```python
from build123d import *

# Parameters (mm, degrees)
SKETCH1_W           = 120
SKETCH1_H           = 200
BOSS_EXTRUDE1_DEPTH = 20
SKETCH2_W           = 120
SKETCH2_H           = 70
BOSS_EXTRUDE2_DEPTH = 15
SKETCH3_R           = 15
CUT_EXTRUDE1_DEPTH  = 119.321595662
FILLET1_R           = 40
CHAMFER1_SIZE       = 7
SHELL2_T            = -5


with BuildPart() as part:
    # Sketch1 → Boss-Extrude1 (new body)
    with BuildSketch(Plane.XY):
        Rectangle(SKETCH1_W, SKETCH1_H)
    extrude(amount=BOSS_EXTRUDE1_DEPTH)

    # Sketch2 → Boss-Extrude2 (add)
    with BuildSketch(Plane.XY.offset(20)):
        with Locations((0, -65)):
            Rectangle(SKETCH2_W, SKETCH2_H)
    extrude(amount=BOSS_EXTRUDE2_DEPTH)

    # Sketch3 → Cut-Extrude1 (cut, through all)
    with BuildSketch(Plane.XY.offset(20)):
        with Locations((-30, 70)):
            Circle(SKETCH3_R)
    extrude(amount=-CUT_EXTRUDE1_DEPTH, mode=Mode.SUBTRACT)

    # Fillet1
    fillet1_edges = [part.edges().sort_by_distance(p)[0] for p in [
        (60, -30, 27.5),
        (60, 100, 10),
    ]]
    fillet(fillet1_edges, radius=FILLET1_R)

    # Chamfer1
    chamfer1_edges = [part.edges().sort_by_distance(p)[0] for p in [
        (60, -5, 20),
        (60, -85, 35),
        (-20, -30, 35),
        (48.284271247, -41.715728753, 35),
        (-20, 100, 20),
        (48.284271247, 88.284271247, 20),
    ]]
    chamfer(chamfer1_edges, length=CHAMFER1_SIZE)

    # Shell2
    shell2_openings = [part.faces().sort_by_distance(p)[0] for p in [
        (0.159993916, -3.518488273, 0),
        (-0.338362671, -100, 17.411008662),
    ]]
    offset(amount=SHELL2_T, openings=shell2_openings, kind=Kind.INTERSECTION)


solid = part.part
```
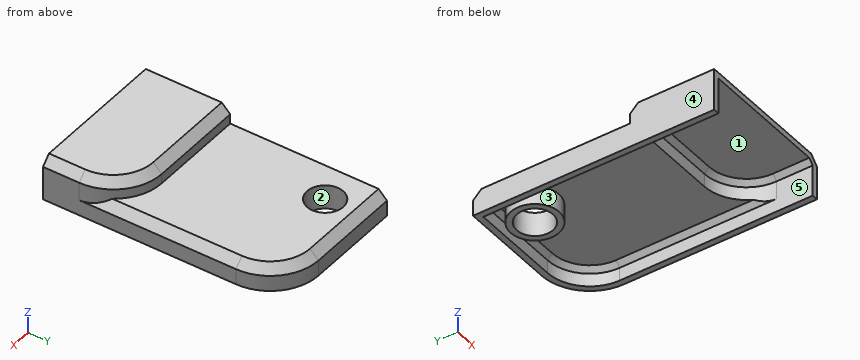
Input: part model. Units: mm. Frame: model coordinates. Face numbers are marked on the shaded views. A direction names the side the tool comes from. Coordinates: 2 decimals unless noted, no trailing zeros. Loops run counter-clockwise (first coordinate to the right, second up) from the corner with the lowest first, then second, coordinate; pieces in that order, holes last. Notation, with made-up numbers: (46.25, 52.5) - (105.25, 52.5) arc R27 cw to (105.25, 89.5) - close; hole circle Ø1 at (83, -21). An arc over 180 degrees is marked (long way). Answer in a Markdown table with one row per item.
(1) Cut plane A-A on x = -30. Output: boundary loops of the cut face in (y, z), plus the area to 3 significant figures.
Model answer:
| item | result |
|---|---|
| outline | (-100, 30) - (-39.07, 30) - (-35, 25.93) - (-35, 15) - (50, 15) - (50, 0) - (55, 0) - (55, 20) - (-30, 20) - (-30, 28) - (-37, 35) - (-100, 35) - close; (85, 0) - (90, 0) - (90, 15) - (90.93, 15) - (95, 10.93) - (95, 0) - (100, 0) - (100, 13) - (93, 20) - (85, 20) - close |
| area | 1,120 mm² |
(2) Set-up query: the marked faces 3, 4 and 5. Return all of +Z, -Z, +X, -X, +Y, -Y with unobstructed straight access to the full face (end or side cutting, diameter ignored); none if empty.
Model answer:
| item | result |
|---|---|
| face 3 | -Z |
| face 4 | +Z, -Z, -X, +Y, -Y |
| face 5 | -Z, -Y |
(3) Pin query (flat end, axial travel): P1, Ø6, axis at x = -2.5, z = 16.5, coming from the +Y side; P2, Ø12, axis at x = -23.5, z = 22, coming from the -Y side; P3, Ø4, axis at x = -11.5, z = 24, coming from the +Y side; P4, Ø9, axis at y = 40.5, z = 15.5, coming from the +X side. Return the tip coordinate at first contact, or that it passes through.
Model answer:
| item | result |
|---|---|
| P1 | stops at y = 99.5 |
| P2 | stops at y = -37.07 |
| P3 | stops at y = -30 |
| P4 | stops at x = 60 |
(4) Cut plane B-B on z = 23.5. Output: boundary loops of the cut face in (x, y).
Model answer:
| item | result |
|---|---|
| outline | (-60, -100) - (-55, -100) - (-55, -35) - (20, -35) arc R35 cw to (55, -70) - (55, -100) - (60, -100) - (60, -70) arc R40 ccw to (20, -30) - (-60, -30) - close |
(5) Cut plane C-C on x = -7. Output: boundary loops of the cut face in (y, z).
Model answer:
| item | result |
|---|---|
| outline | (-100, 30) - (-39.07, 30) - (-35, 25.93) - (-35, 15) - (90.93, 15) - (95, 10.93) - (95, 0) - (100, 0) - (100, 13) - (93, 20) - (-30, 20) - (-30, 28) - (-37, 35) - (-100, 35) - close |
(6) Cut plane D-D on z = 32.5. Output: boundary loops of the cut face in (x, y).
Model answer:
| item | result |
|---|---|
| outline | (-60, -100) - (55.5, -100) - (55.5, -70) arc R35.5 ccw to (20, -34.5) - (-60, -34.5) - close |
(7) Mould query, pull axis Y, two halves, no side actions, for the marked faces 1 and 2. Classes: pulls with the +Y half, pulls with the -Y half, needs draft (parallel to the pull), parting line crosses it, or undercut.
Model answer:
| item | result |
|---|---|
| face 1 | needs draft |
| face 2 | undercut |
(8) Material intervals for L1, parallel to Y at x = -30, z = 8; L2, parallel to X at y = 57, z = 14.5; L3, parallel to X at y = -71.5, z = 22, sorted ascending. Write a range as from..to.
Model answer:
| item | result |
|---|---|
| L1 | y = 50..55, 85..90, 95..100 |
| L2 | x = -60..-55, -45.2..-37.48, -22.52..-14.8, 51.43..58.5 |
| L3 | x = -60..-55, 55..60 |
